Read the model definition and answer for the solid it produces. Units are mm, in the model's axes. Give positions to 0.01 mm unless a question says otherwise; leave off trailing zeros. Loops run counter-clockwise (first coordinate to the right, second up) from the corner with the lowest first, then second, coordinate; pieces in that order, holes last. Notation, with made-up numbers: (11.25, -12.75) - (44.25, -12.75) arc R37 cw to (44.25, 24.25) - close; hole circle Ø2 at (33.5, 21.25). An arc over 180 degrees is marked (long way). Put each result on its own line as item: value. Start each with the question number.
1. Consider L1, parallel to Y at x = 51, z = 15; L2, parallel to Z at x = 54, y = -19.05; L3, parallel to Z at x = -2, y = 62.5. Determine where each line is inside the solid, lowest interval first. Write a range as from..to.
2. A cutting plane is placed at B-B, the plane z = 12.7. Count the separate pieces of the cut face and the enclosed holes in it, plus the area to 3 significant figures.
3. A cutting plane is placed at A-A, the plane y = -11.5. Determine the outline of the cut face in (x, z), plus the area to 3 significant figures.
4. Given pin 1 Ø1.4 at (y, z) = (117, 1.5) entering from +X; pin 2 Ø10 at (y, z) = (-87.5, 16) entering from +X; pin 3 Ø0.5 at (x, y) = (14.5, 120) entering from -Z; pin 4 Ø1.5 at (x, y) = (-37, 67) entering from -Z, each flat-ended and moving along its own axis, determine where each tip first touches the part or whether it passes through.
5. A cutting plane is placed at C-C, the plane y = -101.6. Determine the outline of the cut face in (x, z).
```python
from build123d import *

# Parameters (mm, degrees)
F0_R      = 1.5875
F1_DEPTH  = 6.35
F2_W      = 6.35
F2_H      = 25.4
F3_DEPTH  = 15.24
F5_D      = 10.414
F8_W      = 2.31775
F8_H      = 1.27
F9_DEPTH  = 6.35
F11_W     = 2.31775
F11_H     = 1.27
F12_DEPTH = 6.35
F13_R     = 0.508
F15_DEPTH = 25.4


with BuildPart() as f1:
    # F0 (on Top) → F1 (new body)
    with BuildSketch(Plane.XY):
        Polygon((69.85, 114.3), (-69.85, 114.3), (-69.85, -114.3), (-44.45, -114.3), (-44.45, -107.95), (-44.45, -38.1), (-20.32, -38.1), (-20.32, 19.05), (0, 19.05), (0, 6.35), (44.45, 6.35), (44.45, -38.1), (44.45, -88.9), (44.45, -95.25), (44.45, -114.3), (69.85, -114.3), align=None)
        with Locations((-52.91582, 53.975)):
            Circle(F0_R, mode=Mode.SUBTRACT)
        with Locations((-44.45, 53.975)):
            Circle(F0_R, mode=Mode.SUBTRACT)
        with Locations((-12.7, 46.0375)):
            Circle(F0_R, mode=Mode.SUBTRACT)
        with Locations((-12.7, 68.2625)):
            Circle(F0_R, mode=Mode.SUBTRACT)
    extrude(amount=F1_DEPTH)

    # F2 (on face) → F3 (join)
    with BuildSketch(Plane.XY.offset(6.35)):
        with Locations((-53.975, -101.6)):
            Rectangle(F2_W, F2_H)
        with Locations((53.975, -101.6)):
            Rectangle(F2_W, F2_H)
        with Locations((-53.975, -19.05)):
            Rectangle(F2_W, F2_H)
        with Locations((53.975, -19.05)):
            Rectangle(F2_W, F2_H)
    extrude(amount=F3_DEPTH)

    # F5 (through all)
    with Locations(Plane.YZ.offset(57.15)):
        with Locations((-101.6, 12.7), (-19.05, 12.7)):
            Hole(F5_D / 2)

    # F8 (on offset) → F9 (join)
    with BuildSketch(Plane.YZ.offset(12.7)):
        with Locations((120.094375, 4.0005)):
            Rectangle(F8_W, F8_H)
        Polygon((118.9355, 3.3655), (118.9355, 4.6355), (116.61775, 4.6355), (116.61775, 3.175), (114.3, 3.175), (114.3, 0), (118.9355, 0), align=None)
    extrude(amount=F9_DEPTH)

    # F11 (on offset) → F12 (join)
    with BuildSketch(Plane.YZ.offset(-12.7)):
        with Locations((120.094375, 4.0005)):
            Rectangle(F11_W, F11_H)
        Polygon((118.9355, 3.3655), (118.9355, 4.6355), (116.61775, 4.6355), (116.61775, 3.175), (114.3, 3.175), (114.3, 0), (118.9355, 0), align=None)
    extrude(amount=-F12_DEPTH)

    # F13
    f13_edges = [f1.edges().sort_by_distance(p)[0] for p in [
        (15.875, 121.25325, 3.3655),
        (-15.875, 121.25325, 3.3655),
        (-15.875, 116.61775, 4.6355),
        (15.875, 116.61775, 4.6355),
    ]]
    fillet(f13_edges, radius=F13_R)

    # F14 (on face) → F15 (cut)
    with BuildSketch(Plane.XY.offset(6.35)):
        Polygon((-49.2903768363, -40.005), (-65.0113, -40.005), (-65.0113, -55.7259231637), align=None)
        Polygon((-49.2903768363, -58.42), (-49.2903768363, -42.6990768363), (-65.0113, -58.42), align=None)
        Polygon((-49.2903768363, -62.23), (-65.0113, -62.23), (-49.2903768363, -77.9509231637), align=None)
        Polygon((-65.0113, -64.9240768363), (-65.0113, -80.645), (-49.2903768363, -80.645), align=None)
        Polygon((65.0113, -64.9240768363), (49.2903768363, -80.645), (65.0113, -80.645), align=None)
        Polygon((49.2903768363, -77.9509231637), (65.0113, -62.23), (49.2903768363, -62.23), align=None)
        Polygon((65.0113, -58.42), (49.2903768363, -42.6990768363), (49.2903768363, -58.42), align=None)
        Polygon((49.2903768363, -40.005), (65.0113, -55.7259231637), (65.0113, -40.005), align=None)
    extrude(amount=-F15_DEPTH, mode=Mode.SUBTRACT)


solid = f1.part
```
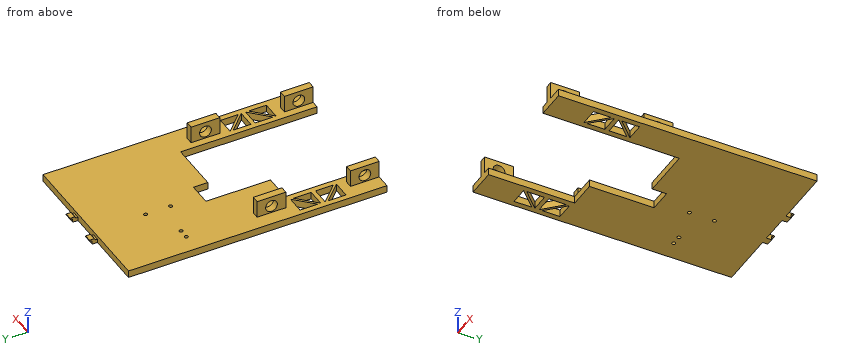
Return value:
1. L1: y = -114.3..-106.27, -96.93..-88.9, -31.75..-23.72, -14.38..-6.35
1. L2: z = 0..7.49, 17.91..21.59
1. L3: z = 0..6.35
2. separate pieces: 8
2. enclosed holes: 0
2. area: 381 mm2
3. outline: (-69.85, 0) - (-20.32, 0) - (-20.32, 6.35) - (-50.8, 6.35) - (-50.8, 21.59) - (-57.15, 21.59) - (-57.15, 6.35) - (-69.85, 6.35) - close; (44.45, 0) - (69.85, 0) - (69.85, 6.35) - (57.15, 6.35) - (57.15, 21.59) - (50.8, 21.59) - (50.8, 6.35) - (44.45, 6.35) - close
3. area: 669 mm2
4. pin 1: stops at x = 19.05
4. pin 2: stops at x = 57.15
4. pin 3: stops at z = 3.37
4. pin 4: stops at z = 0
5. outline: (-69.85, 0) - (-44.45, 0) - (-44.45, 6.35) - (-50.8, 6.35) - (-50.8, 7.49) - (-57.15, 7.49) - (-57.15, 6.35) - (-69.85, 6.35) - close; (-57.15, 17.91) - (-50.8, 17.91) - (-50.8, 21.59) - (-57.15, 21.59) - close; (44.45, 0) - (69.85, 0) - (69.85, 6.35) - (57.15, 6.35) - (57.15, 7.49) - (50.8, 7.49) - (50.8, 6.35) - (44.45, 6.35) - close; (50.8, 17.91) - (57.15, 17.91) - (57.15, 21.59) - (50.8, 21.59) - close
